Work out the finished part from the listing and answer in its coordinate system (mm). A direction names the side the tool comes from. Round coordinates to 2 decimals unless told otherwise and drop trailing zeros. Loops run counter-clockwise (first coordinate to the right, second up) from the corner with the lowest first, then second, coordinate; pieces in that order, holes last.
from build123d import *

# Parameters (mm, degrees)
F0_W     = 52.5484979153
F0_H     = 51.326431334
F1_DEPTH = 50
F2_DEPTH = 35
F3_T     = -5
F4_R     = 10
F5_R     = 10


with BuildPart() as f1:
    # F0 (on Front) → F1 (new body)
    with BuildSketch(Plane.XZ):
        with Locations((26.2742489576, 25.663215667)):
            Rectangle(F0_W, F0_H)
    extrude(amount=F1_DEPTH)

    # F2 (add): a face of the model
    f2_faces = [f1.faces().sort_by_distance(p)[0] for p in [
        (26.2742489576, -25, 51.326431334),
    ]]
    extrude(f2_faces, amount=F2_DEPTH)

    # F3
    f3_openings = [f1.faces().sort_by_distance(p)[0] for p in [
        (26.274249, -50, 43.163216),
    ]]
    offset(amount=F3_T, openings=f3_openings)

    # F4
    f4_edges = [f1.edges().sort_by_distance(p)[0] for p in [
        (0, -25, 0),
        (52.548498, -25, 0),
        (0, -25, 86.326431),
        (52.548498, -25, 86.326431),
    ]]
    fillet(f4_edges, radius=F4_R)

    # F5
    f5_edges = [f1.edges().sort_by_distance(p)[0] for p in [
        (5, -27.5, 5),
        (47.548498, -27.5, 5),
        (47.548498, -27.5, 81.326431),
        (5, -27.5, 81.326431),
    ]]
    fillet(f5_edges, radius=F5_R)


solid = f1.part
Item 1: Each of these flat-tipped pins is pushed along its axis until it touches: P1, Ø10, axis at y = -9, z = 9.5, coming from the +X side; P2, Ø21.5, axis at x = 26, z = 29.5, coming from the -Y side; P3, Ø1.5, axis at x = 47, y = -17, coming from the +Z side. Where does it stop, or does it pass through?
Item 2: Section A-A, the plane y = -41 is taken. Give the vertices of the cut face in (x, z), plus the area to 3 significant figures.
Item 3: Straight lines are drawn through the part: line 1 (Z direction, x = 29.5, y = -24.5); line 2 (X direction, y = -34.5, z = 51); line 3 (Y direction, x = 47.5, z = 43.5). For each, find the intervals that lie inside material, in ascending order.
Item 4: For faces 1 (the face through (8.007, -27.185, 78.475)), 2 (the face through (49.54, -25.35, 2.85)), determine the directions among +Z, -Z, +X, -X, +Y, -Y from which every point of the face is accessible in a straight line to the end or side of a thin tool.
Item 5: Section B-B, the plane x = 29 is taken. Give the vertices of the cut face in (y, z), plus the area to 3 significant figures.
Item 6: Section C-C, the plane z = 51 is taken. Give the vertices of the cut face in (x, y), plus the area to 3 significant figures.
Answer below:
1. P1: stops at x = 52.55
1. P2: stops at y = -5
1. P3: stops at z = 85.62
2. outline: (0, 10) arc R10 ccw to (10, 0) - (42.55, 0) arc R10 ccw to (52.55, 10) - (52.55, 76.33) arc R10 ccw to (42.55, 86.33) - (10, 86.33) arc R10 ccw to (0, 76.33) - close; hole (5, 15) arc R10 ccw to (15, 5) - (37.55, 5) arc R10 ccw to (47.55, 15) - (47.55, 71.33) arc R10 ccw to (37.55, 81.33) - (15, 81.33) arc R10 ccw to (5, 71.33) - close
2. area: 1,290 mm2
3. line 1: z = 0 to 5, 81.33 to 86.33
3. line 2: x = 0 to 5, 47.55 to 52.55
3. line 3: y = -5 to 0
4. face 1: -Y
4. face 2: -Z, +X, +Y, -Y
5. outline: (-50, 0) - (0, 0) - (0, 86.33) - (-50, 86.33) - (-50, 81.33) - (-5, 81.33) - (-5, 5) - (-50, 5) - close
5. area: 882 mm2
6. outline: (0, -50) - (5, -50) - (5, -5) - (47.55, -5) - (47.55, -50) - (52.55, -50) - (52.55, 0) - (0, 0) - close
6. area: 713 mm2
